Build history of the part. All positions in model axes, mm. Face numbers are marked on the shaded views. A direction names the side the tool comes from. Give positions to 0.01 mm unless a question says otherwise; leave off trailing zeros. Loops run counter-clockwise (first coordinate to the right, second up) from the corner with the lowest first, then second, coordinate; pieces in that order, holes last. Notation, with made-up numbers: (39, 59) -> (49, 59) arc R17 ccw to (49, 85) -> close; hole circle Ø4 at (53.25, 42). An arc over 180 degrees is marked (long way). Answer as a JSON object with one key per item and string values. Group by question number.
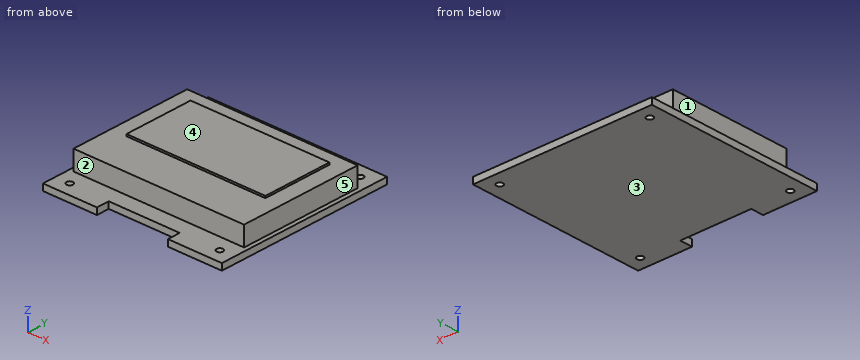
from build123d import *

# Parameters (mm, degrees)
ESQUISSE1_R        = 0.5
BOSS_EXTRU_1_DEPTH = 1
ESQUISSE2_W        = 26.7
ESQUISSE2_H        = 19.26
BOSS_EXTRU_2_DEPTH = 3
ESQUISSE4_W        = 21.744
ESQUISSE4_H        = 10.864
BOSS_EXTRU_3_DEPTH = 0.3


with BuildPart() as part:
    # Esquisse1 → Boss.-Extru.1 (new body)
    with BuildSketch(Plane.XY):
        Polygon((-10.934549339, 15.65387995), (17.065450661, 15.65387995), (17.065450661, -12.34612005), (8.625947463, -12.34612005), (8.625947463, -10.34612005), (3.065450661, -10.34612005), (-2.495046141, -10.34612005), (-2.495046141, -12.34612005), (-10.934549339, -12.34612005), align=None)
        with Locations((-8.684549339, -10.24612005)):
            Circle(ESQUISSE1_R, mode=Mode.SUBTRACT)
        with Locations((-8.684549339, 13.55387995)):
            Circle(ESQUISSE1_R, mode=Mode.SUBTRACT)
        with Locations((14.815450661, 13.55387995)):
            Circle(ESQUISSE1_R, mode=Mode.SUBTRACT)
        with Locations((14.815450661, -10.24612005)):
            Circle(ESQUISSE1_R, mode=Mode.SUBTRACT)
    extrude(amount=BOSS_EXTRU_1_DEPTH)

    # Esquisse2 → Boss.-Extru.2 (add)
    with BuildSketch(Plane.XY.offset(1)):
        with Locations((3.065450661, 1.75387995)):
            Rectangle(ESQUISSE2_W, ESQUISSE2_H)
    extrude(amount=BOSS_EXTRU_2_DEPTH)

    # Esquisse4 → Boss.-Extru.3 (add)
    with BuildSketch(Plane.XY.offset(4)):
        with Locations((3.065450661, 3.85187995)):
            Rectangle(ESQUISSE4_W, ESQUISSE4_H)
    extrude(amount=BOSS_EXTRU_3_DEPTH)


solid = part.part
(1) 3-axis set-ups, long thin cutter, end or side, ignore diameter. For the marked faces 1 and 2: which of +Z, -Z, +X, -X, +Y, -Y reach the whole face in a straight line?
(2) Saw through at D-D on x = 1. List the corners of the cut face in (y, z).
(3) Pull direction Z, two halves, no side cores. Call the marked faces 3, 4 and 5: pulls with the +Z half, pulls with the -Z half, needs draft (parallel to the pull), parting line crosses it, or undercut.
(4) Probe line 1 along Z through (x, y) = (-0.75, 11.25); line 2 along Y through (x, z) = (13.25, 2.3); line 3 along X through (y, z) = (-7.5, 2.05). List the from-to ranges inside material, lowest first. Write a range as [from, to].
(5) Saw through at A-A on x = -5.75. List the corners of the cut face in (y, z), plus the area to 3 significant figures.
(6) Saw through at C-C on z = 2.55. List the corners of the cut face in (x, y), plus the area to 3 significant figures.
(7) Saw through at B-B on y = -2.75. List the corners of the cut face in (x, z).
(8) Pin check, flat tips, straight feed: pin 1 (0.9 mm diameter, centred on x = 5.5, z = 3, fed in from +Y); pin 2 (1.5 mm diameter, centred on x = 13, z = 3.5, fed in from -Y); pin 3 (1.5 mm diameter, centred on y = 1, z = 3, fed in from +X). Stop position of each tip, or through.
Calculated:
{
 "1": {"face 1": "+Z, -X, +Y, -Y", "face 2": "+Z, +X, -X, -Y"},
 "2": {"outline": "(-10.35, 0) -> (15.65, 0) -> (15.65, 1) -> (11.38, 1) -> (11.38, 4) -> (9.28, 4) -> (9.28, 4.3) -> (-1.58, 4.3) -> (-1.58, 4) -> (-7.88, 4) -> (-7.88, 1) -> (-10.35, 1) -> close"},
 "3": {"face 3": "pulls with the -Z half", "face 4": "pulls with the +Z half", "face 5": "needs draft"},
 "4": {"line 1": "z = [0, 4]", "line 2": "y = [-7.88, 11.38]", "line 3": "x = [-10.28, 16.42]"},
 "5": {"outline": "(-12.35, 0) -> (15.65, 0) -> (15.65, 1) -> (11.38, 1) -> (11.38, 4) -> (9.28, 4) -> (9.28, 4.3) -> (-1.58, 4.3) -> (-1.58, 4) -> (-7.88, 4) -> (-7.88, 1) -> (-12.35, 1) -> close", "area": "89.0 mm^2"},
 "6": {"outline": "(-10.28, -7.88) -> (16.42, -7.88) -> (16.42, 11.38) -> (-10.28, 11.38) -> close", "area": "514 mm^2"},
 "7": {"outline": "(-10.93, 0) -> (17.07, 0) -> (17.07, 1) -> (16.42, 1) -> (16.42, 4) -> (-10.28, 4) -> (-10.28, 1) -> (-10.93, 1) -> close"},
 "8": {"pin 1": "stops at y = 11.38", "pin 2": "stops at y = -7.88", "pin 3": "stops at x = 16.42"}
}
